Autodesk Inventor part; units mm, degrees
ref_plane "Work Plane1" through (0, 0, -15) normal (0, 0, 1) x (1, 0, 0)
ref_plane "YZ Plane" through (0, 0, 0) normal (1, 0, 0) x (0, 1, 0)
ref_plane "XZ Plane" through (0, 0, 0) normal (0, 1, 0) x (-1, 0, 0)
sketch "Sketch1" plane through (0, 0, 0) normal (0, 0, 1) x (1, 0, 0)
  line L0 (0, 0) -> (25, 0)
  line L1 (25, 0) -> (25, 40)
  line L2 (25, 40) -> (0, 40)
  line L3 (0, 40) -> (0, 0)
  dimension "d1" = 25
  dimension "d2" = 40
  dimension "d3" = 25
extrude "Extrusion1" add sketch "Sketch1" against normal blind 30
sketch "Sketch2" plane through (25, 0, 0) normal (1, 0, 0) x (0, 0, -1)
  line L0 (0, 0) -> (30, 0)
  circle A0 centre (15, 6.56) radius 2.46
extrude "Extrusion2" cut sketch "Sketch2" against normal blind 30
sketch "Sketch3" plane through (0, 0, 0) normal (-1, 0, 0) x (0, 0, 1)
  line L0 (0, 0) -> (-30, 0)
  line L1 (-25.05, 0) -> (-4.95, 0)
  line L2 (-4.95, 0) -> (-4.95, 33.12)
  line L3 (-4.95, 33.12) -> (-25.05, 33.12)
  line L4 (-25.05, 33.12) -> (-25.05, 0)
  dimension "d11" = 20.1
extrude "Extrusion3" cut sketch "Sketch3" against normal blind 20
sketch "Sketch4" plane through (0, 0, 0) normal (0, -1, 0) x (1, 0, 0)
  line L0 (20, -4.95) -> (20, -25.05)
  line L1 (20, -15) -> (25, -15)
  line L2 (25, 0) -> (25, -30)
  line L3 (20, -8.025) -> (25, -8.025)
  line L4 (25, -8.025) -> (25, -21.975)
  line L5 (25, -21.975) -> (20, -21.975)
  line L6 (20, -21.975) -> (20, -8.025)
  line L7 (20, -8.025) -> (25, -21.975) construction
  line L8 (25, -8.025) -> (20, -21.975) construction
  line L9 (25, -12.54) -> (25, -17.46)
  point P0 (0, 0)
  point P1 (22.5, -15)
  dimension "d14" = 13.95
extrude "Extrusion4" add sketch "Sketch4" along normal blind 15
sketch "Sketch5" plane through (20, 0, 0) normal (-1, 0, 0) x (0, 0, 1)
  circle A0 centre (-15, 6.56) radius 2.46
  circle A1 centre (-15, 6.56) radius 4.7025
  circle A2 centre (-15, 6.56) radius 2.46
  circle A3 centre (-15, 6.56) radius 2.46
  point P0 (0, 0)
  dimension "d17" = 9.405
extrude "Extrusion5" cut sketch "Sketch5" against normal blind 2.1
sketch "Sketch6" plane through (25, 0, 0) normal (1, 0, 0) x (0, 0, -1)
  circle A0 centre (15, 6.56) radius 4.7025
  line L0 (15, 6.56) -> (15, 23.56)
  circle A1 centre (15, 23.56) radius 2.46
  point P0 (0, 0)
  dimension "d20" = 17
  dimension "d21" = 4.92
extrude "Extrusion6" cut sketch "Sketch6" against normal blind 10 contours A1
sketch "Sketch7" plane through (20, 0, 0) normal (-1, 0, 0) x (0, 0, 1)
  circle A0 centre (-15, 23.56) radius 2.46
  circle A1 centre (-15, 23.56) radius 4.7025
  point P0 (0, 0)
  dimension "d24" = 9.405
extrude "Extrusion7" cut sketch "Sketch7" against normal blind 2.1
sketch "Sketch9" plane through (25, 0, 0) normal (1, 0, 0) x (0, 0, -1)
  circle A0 centre (15, 6.56) radius 2.46
  circle A1 centre (15, 6.56) radius 2.46
  circle A2 centre (15, 23.56) radius 2.46
  circle A3 centre (15, 23.56) radius 2.46
  line L0 (30, 40) -> (30, 0)
  line L1 (30, 0) -> (30, 40)
  line L2 (30, 40) -> (0, 40)
  line L3 (0, 40) -> (0, 0)
  line L4 (0, 0) -> (8.025, 0)
  line L5 (21.975, 0) -> (21.975, -15)
  line L6 (21.975, -15) -> (8.025, -15)
  line L7 (8.025, -15) -> (8.025, 0)
  line L8 (0, 0) -> (8.025, 0)
  line L9 (21.975, 0) -> (30, 0)
extrude "Extrusion8" add sketch "Sketch9" along normal blind 5
sketch "Sketch10" plane through (0, 40, 0) normal (0, 1, 0) x (1, 0, 0)
  line L0 (0, 30) -> (30, 30)
  line L1 (30, 0) -> (0, 0)
  line L2 (0, 30) -> (30, 30)
  line L3 (30, 30) -> (30, 0)
  line L4 (30, 0) -> (0, 0)
  line L5 (0, 0) -> (0, 30)
extrude "Extrusion9" add sketch "Sketch10" along normal blind 30
sketch "Sketch12" plane through (30, 0, 0) normal (1, 0, 0) x (0, 0, -1)
  circle A0 centre (15, 6.56) radius 2.46
  line L0 (15, 6.56) -> (15, 15.06)
  circle A1 centre (15, 15.06) radius 2.525
  point P0 (0, 0)
  dimension "d31" = 8.5
  dimension "d33" = 5.05
extrude "Extrusion10" cut sketch "Sketch12" against normal blind 30 contours A1
sketch "Sketch14" plane through (0, 0, 0) normal (0, 0, 1) x (1, 0, 0)
  line L0 (30, 70) -> (0, 70)
  line L1 (0, 70) -> (0, 85)
  line L2 (30, 0) -> (30, 70)
  line L3 (30, 113) -> (30, 70)
  line L4 (30, 105) -> (30, 100)
  line L5 (-12, 128) -> (15, 128)
  line L6 (-8, 126) -> (-12, 128)
  line L7 (-8, 126) -> (-4, 114)
  line L8 (-8, 102) -> (-12, 100)
  line L9 (-8, 102) -> (-4, 114)
  line L10 (30, 113) -> (15, 128)
  line L11 (0, 100) -> (-12, 100)
  line L12 (0, 100) -> (0, 85)
  point P0 (0, 0)
  dimension "d69" = 28
  dimension "d74" = 12
extrude "Extrusion12" add sketch "Sketch14" against normal blind 30
sketch "Sketch15" plane through (0, 0, -25.05) normal (-1, 0, 0) x (0, 0, 1)
  line L0 (0, 33.12) -> (20.1, 33.12)
  line L1 (20.1, 33.12) -> (20.1, 0)
  line L2 (0, 33.12) -> (20.1, 33.12)
  line L3 (20.1, 33.12) -> (20.1, 31.1)
  line L4 (20.1, 31.1) -> (0, 31.1)
  line L5 (0, 31.1) -> (0, 33.12)
  point P0 (25.05, 0)
  dimension "d57" = 2.02
extrude "Extrusion13" add sketch "Sketch15" against normal blind 20
sketch "Sketch21" plane through (0, 0, 0) normal (0, 0, 1) x (1, 0, 0)
  line L0 (0, 100) -> (-12, 100)
  line L1 (0, 100) -> (-12, 100)
  line L2 (-12, 100) -> (-8, 102)
  line L3 (-12, 100) -> (-8, 102)
  line L4 (-8, 102) -> (-4, 114)
  line L5 (-8, 102) -> (-4, 114)
  line L6 (-4, 114) -> (-8, 126)
  line L7 (-4, 114) -> (-8, 126)
  line L8 (-8, 126) -> (-12, 128)
  line L9 (-8, 126) -> (-12, 128)
  line L10 (-12, 128) -> (15, 128)
  line L11 (-12, 128) -> (15, 128)
  line L12 (15, 128) -> (30, 113)
  line L13 (15, 128) -> (30, 113)
  line L14 (30, 113) -> (30, 93)
  line L15 (30, 0) -> (30, 113)
  line L16 (30, 93) -> (0, 93)
  line L17 (0, 93) -> (0, 100)
  point P0 (0, 0)
  dimension "d75" = 20
  dimension "d76" = 30
extrude "Extrusion14" add sketch "Sketch21" along normal blind 45
ref_plane "Work Plane1" through (0, 0, -15) normal (0, 0, 1) x (1, 0, 0)
mirror "Mirror1" about plane through (0, 0, -15) normal (0, 0, 1) of "Extrusion14"
properties part number "rec_b_24mm_x_120mm"
Design review of the part built by this model. Coordinates are the model's own, in mm. A direction names the side the tool comes from. Coordinates: 2 decimals unless noted, no trailing zeros. Loops run counter-clockwise (first coordinate to the right, second up) from the corner with the lowest first, then second, coordinate; pieces in that order, holes last.
Q1. To check wall thickness, follow line 1 (Z direction, x = 24, y = 23.56); line 2 (Z direction, x = 21, y = 6); line 3 (Y direction, x = 21, z = -15) (1 decimal). State the ranges of each line that lie inside material, in increasing order.
Reported:
line 1: z = -30 to -17.46, -12.54 to 0
line 2: z = -30 to -19.67, -10.33 to 0
line 3: y = -15 to 1.9, 11.3 to 12.5, 17.6 to 18.9, 28.3 to 122
Q2. For pin 1 (4 mm diameter, centred on x = 8.5, y = 79, fed in from +Z); pin 2 (7.5 mm diameter, centred on y = 6.56, z = -15, fed in from -X); pin 3 (22 mm diameter, centred on x = 8, y = 18, fed in from -Z); pin 4 (12 mm diameter, centred on y = 23.56, z = -15, fed in from +X), all flat-tipped, find the tip position at first contact; note any pin that passes through.
Reported:
pin 1: stops at z = 0
pin 2: stops at x = 22.1
pin 3: stops at z = -30
pin 4: stops at x = 30
Q3. We need section B-B on y = 23.56. State the section outline as (x, z) points.
Reported:
outline: (0, -30) - (30, -30) - (30, -17.46) - (22.1, -17.46) - (22.1, -19.7) - (20, -19.7) - (20, -25.05) - (0, -25.05) - close; (0, -4.95) - (20, -4.95) - (20, -10.3) - (22.1, -10.3) - (22.1, -12.54) - (30, -12.54) - (30, 0) - (0, 0) - close
Q4. We need section D-D on x = 5.5. State the section outline as (y, z) points.
Reported:
outline: (0, -30) - (93, -30) - (93, -75) - (128, -75) - (128, 45) - (93, 45) - (93, 0) - (0, 0) - (0, -4.95) - (31.1, -4.95) - (31.1, -25.05) - (0, -25.05) - close
Q5. We need section C-C on x = 24. State the section outline as (y, z) points (3 decimals).
Reported:
outline: (-15, -21.975) - (0, -21.975) - (0, -30) - (93, -30) - (93, -75) - (119, -75) - (119, 45) - (93, 45) - (93, 0) - (0, 0) - (0, -8.025) - (-15, -8.025) - close; hole circle Ø4.92 at (6.56, -15); hole circle Ø5.05 at (15.06, -15); hole circle Ø4.92 at (23.56, -15)
Q6. We need section A-A on z = -15. State how many separate pieces and enclosed holes the cut face has, and give its area (3 significant figures).
Reported:
separate pieces: 4
enclosed holes: 0
area: 3,270 mm2
Q7. Tool access review of faces 1 (the face through (21.035, 27.525, -12.472)), 2 (the face through (-6, 120, -14)), 3 (the face through (25, -8, -8.025)), 4 (the face through (25.995, 7.502, -17.272)): name each direction out of +Z, -Z, +X, -X, +Y, -Y from which nothing blocks a thin tool from reaching the whole face with its end or side.
Reported:
face 1: -X
face 2: +Z, -Z, -X
face 3: +Z, +X, -X, -Y
face 4: +X, -X
Q8. The part is to be moulded in two halves that separate along Z. For faces 5 (the face through (20, 8, -20)), 6 (the face through (0, 62, -14)), 7 (the face through (25, -7, -21.975)), 8 (the face through (10, 15, -4.95)), say which applies: +Z half, -Z half, draft (parallel to the pull), parting line (faces both ways), or undercut.
Reported:
face 5: undercut
face 6: draft
face 7: -Z half
face 8: undercut
